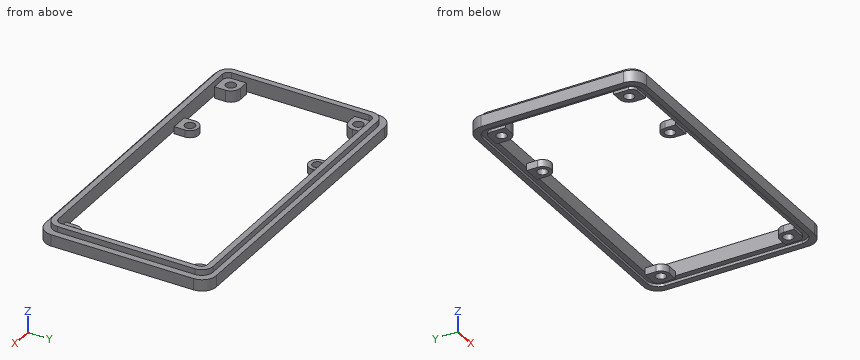
from build123d import *

# Parameters (mm, degrees)
F1_DEPTH = 6
F2_DEPTH = 4
F0_R     = 1.75
F3_DEPTH = 2.5
F4_DEPTH = 4
F5_DEPTH = 1


with BuildPart() as f1:
    # F0 (on Top) → F1 (new body)
    with BuildSketch(Plane.XY):
        with BuildLine():
            Line((48.5, 28), (-48.5, 28))
            ThreePointArc((-48.5, 28), (-51.328427, 26.828427), (-52.5, 24))
            Line((-52.5, 24), (-52.5, -24))
            ThreePointArc((-52.5, -24), (-51.328427, -26.828427), (-48.5, -28))
            Line((-48.5, -28), (48.5, -28))
            ThreePointArc((48.5, -28), (51.328427, -26.828427), (52.5, -24))
            Line((52.5, -24), (52.5, 24))
            ThreePointArc((52.5, 24), (51.328427, 26.828427), (48.5, 28))
        make_face()
        with BuildLine():
            ThreePointArc((-50.5, 24), (-49.914214, 25.414214), (-48.5, 26))
            Line((-48.5, 26), (-43.75, 26))
            Line((-43.75, 26), (-25.9, 26))
            Line((-25.9, 26), (-19.9, 26))
            Line((-19.9, 26), (44.1, 26))
            Line((44.1, 26), (48.5, 26))
            ThreePointArc((48.5, 26), (49.914214, 25.414214), (50.5, 24))
            Line((50.5, 24), (50.5, 19.25))
            Line((50.5, 19.25), (50.5, -19.25))
            Line((50.5, -19.25), (50.5, -24))
            ThreePointArc((50.5, -24), (49.914214, -25.414214), (48.5, -26))
            Line((48.5, -26), (44.1, -26))
            Line((44.1, -26), (-19.9, -26))
            Line((-19.9, -26), (-25.9, -26))
            Line((-25.9, -26), (-43.75, -26))
            Line((-43.75, -26), (-48.5, -26))
            ThreePointArc((-48.5, -26), (-49.914214, -25.414214), (-50.5, -24))
            Line((-50.5, -24), (-50.5, -18.9))
            Line((-50.5, -18.9), (-50.5, 18.9))
            Line((-50.5, 18.9), (-50.5, 24))
        make_face(mode=Mode.SUBTRACT)
    extrude(amount=F1_DEPTH)

    # F0 (on Top) → F2 (join)
    with BuildSketch(Plane.XY):
        with BuildLine():
            Line((49.75, 29.875), (-49.75, 29.875))
            ThreePointArc((-49.75, 29.875), (-53.285534, 28.410534), (-54.75, 24.875))
            Line((-54.75, 24.875), (-54.75, -24.875))
            ThreePointArc((-54.75, -24.875), (-53.285534, -28.410534), (-49.75, -29.875))
            Line((-49.75, -29.875), (49.75, -29.875))
            ThreePointArc((49.75, -29.875), (53.285534, -28.410534), (54.75, -24.875))
            Line((54.75, -24.875), (54.75, 24.875))
            ThreePointArc((54.75, 24.875), (53.285534, 28.410534), (49.75, 29.875))
        make_face()
        with BuildLine():
            ThreePointArc((-52.5, 24), (-51.328427, 26.828427), (-48.5, 28))
            Line((-48.5, 28), (48.5, 28))
            ThreePointArc((48.5, 28), (51.328427, 26.828427), (52.5, 24))
            Line((52.5, 24), (52.5, -24))
            ThreePointArc((52.5, -24), (51.328427, -26.828427), (48.5, -28))
            Line((48.5, -28), (-48.5, -28))
            ThreePointArc((-48.5, -28), (-51.328427, -26.828427), (-52.5, -24))
            Line((-52.5, -24), (-52.5, 24))
        make_face(mode=Mode.SUBTRACT)
    extrude(amount=F2_DEPTH)

    # F0 (on Top) → F3 (join)
    with BuildSketch(Plane.XY):
        with BuildLine():
            Line((-19.9, 26), (-25.9, 26))
            Line((-25.9, 26), (-25.9, 22.25))
            ThreePointArc((-25.9, 22.25), (-22.9, 19.25), (-19.9, 22.25))
            Line((-19.9, 22.25), (-19.9, 26))
        make_face()
        with Locations((-22.9, 22.25)):
            Circle(F0_R, mode=Mode.SUBTRACT)
        with BuildLine():
            Line((48.5, 26), (44.1, 26))
            Line((44.1, 26), (44.1, 22.25))
            ThreePointArc((44.1, 22.25), (44.97868, 20.12868), (47.1, 19.25))
            Line((47.1, 19.25), (50.5, 19.25))
            Line((50.5, 19.25), (50.5, 24))
            ThreePointArc((50.5, 24), (49.914214, 25.414214), (48.5, 26))
        make_face()
        with Locations((47.1, 22.25)):
            Circle(F0_R, mode=Mode.SUBTRACT)
        with BuildLine():
            Line((50.5, -24), (50.5, -19.25))
            Line((50.5, -19.25), (47.1, -19.25))
            ThreePointArc((47.1, -19.25), (44.97868, -20.12868), (44.1, -22.25))
            Line((44.1, -22.25), (44.1, -26))
            Line((44.1, -26), (48.5, -26))
            ThreePointArc((48.5, -26), (49.914214, -25.414214), (50.5, -24))
        make_face()
        with Locations((47.1, -22.25)):
            Circle(F0_R, mode=Mode.SUBTRACT)
        with BuildLine():
            Line((-25.9, -22.25), (-25.9, -26))
            Line((-25.9, -26), (-19.9, -26))
            Line((-19.9, -26), (-19.9, -22.25))
            ThreePointArc((-19.9, -22.25), (-22.9, -19.25), (-25.9, -22.25))
        make_face()
        with Locations((-22.9, -22.25)):
            Circle(F0_R, mode=Mode.SUBTRACT)
    extrude(amount=F3_DEPTH)

    # F0 (on Top) → F4 (join)
    with BuildSketch(Plane.XY):
        with BuildLine():
            Line((-43.75, 26), (-48.5, 26))
            ThreePointArc((-48.5, 26), (-49.914214, 25.414214), (-50.5, 24))
            Line((-50.5, 24), (-50.5, 18.9))
            Line((-50.5, 18.9), (-47.1, 18.9))
            ThreePointArc((-47.1, 18.9), (-44.731192, 19.881192), (-43.75, 22.25))
            Line((-43.75, 22.25), (-43.75, 26))
        make_face()
        with Locations((-47.1, 22.25)):
            Circle(F0_R, mode=Mode.SUBTRACT)
        with BuildLine():
            Line((-47.1, -18.9), (-50.5, -18.9))
            Line((-50.5, -18.9), (-50.5, -24))
            ThreePointArc((-50.5, -24), (-49.914214, -25.414214), (-48.5, -26))
            Line((-48.5, -26), (-43.75, -26))
            Line((-43.75, -26), (-43.75, -22.25))
            ThreePointArc((-43.75, -22.25), (-44.731192, -19.881192), (-47.1, -18.9))
        make_face()
        with Locations((-47.1, -22.25)):
            Circle(F0_R, mode=Mode.SUBTRACT)
    extrude(amount=F4_DEPTH)

    # F0 (on Top) → F5 (cut)
    with BuildSketch(Plane.XY):
        with BuildLine():
            Line((48.5, 28), (-48.5, 28))
            ThreePointArc((-48.5, 28), (-51.328427, 26.828427), (-52.5, 24))
            Line((-52.5, 24), (-52.5, -24))
            ThreePointArc((-52.5, -24), (-51.328427, -26.828427), (-48.5, -28))
            Line((-48.5, -28), (48.5, -28))
            ThreePointArc((48.5, -28), (51.328427, -26.828427), (52.5, -24))
            Line((52.5, -24), (52.5, 24))
            ThreePointArc((52.5, 24), (51.328427, 26.828427), (48.5, 28))
        make_face()
        with BuildLine():
            ThreePointArc((-50.5, 24), (-49.914214, 25.414214), (-48.5, 26))
            Line((-48.5, 26), (-43.75, 26))
            Line((-43.75, 26), (-25.9, 26))
            Line((-25.9, 26), (-19.9, 26))
            Line((-19.9, 26), (44.1, 26))
            Line((44.1, 26), (48.5, 26))
            ThreePointArc((48.5, 26), (49.914214, 25.414214), (50.5, 24))
            Line((50.5, 24), (50.5, 19.25))
            Line((50.5, 19.25), (50.5, -19.25))
            Line((50.5, -19.25), (50.5, -24))
            ThreePointArc((50.5, -24), (49.914214, -25.414214), (48.5, -26))
            Line((48.5, -26), (44.1, -26))
            Line((44.1, -26), (-19.9, -26))
            Line((-19.9, -26), (-25.9, -26))
            Line((-25.9, -26), (-43.75, -26))
            Line((-43.75, -26), (-48.5, -26))
            ThreePointArc((-48.5, -26), (-49.914214, -25.414214), (-50.5, -24))
            Line((-50.5, -24), (-50.5, -18.9))
            Line((-50.5, -18.9), (-50.5, 18.9))
            Line((-50.5, 18.9), (-50.5, 24))
        make_face(mode=Mode.SUBTRACT)
    extrude(amount=F5_DEPTH, mode=Mode.SUBTRACT)


solid = f1.part
The listing builds one solid part. Answer for the finished solid, in the listing's coordinates (mm). Round coordinates to 2 decimals unless told otherwise and drop trailing zeros. Write each loop counter-clockwise with the first axis right and the second up, starting at its lowest first coordinate (ties: lowest second). Pieces come first, ordered by that corner, then holes. Notation, with made-up numbers: (-26.5, 42.25) - (-13.5, 42.25) arc R16 ccw to (-13.5, 70.25) - close; hole circle Ø10 at (24.25, 43). An arc over 180 degrees is marked (long way). Use one line per item in the form item = value. Start each with the question number.
Item 1: A cutting plane is placed at C-C (x = -22.9). Give the number of separate pieces and of enclosed holes in the cut face, plus the area to 4 significant figures.
Item 2: A cutting plane is placed at B-B (y = 14.5). Write down the section's boundary in (x, z).
Item 3: Find the intervals of material crossed by line 1 (X direction, y = -22, z = 3.55); line 2 (Y direction, x = 38, z = 3.75) (3 decimals); line 3 (Y direction, x = -50, z = 1.9), in increasing order. Write a range as [from, to].
Item 4: Flat-ended cylindrical pins translate along their axes: pin 1 Ø3.5 at (x, y) = (-46.5, -24) entering from +Z; pin 2 Ø0.6 at (x, z) = (-21.5, 5.5) entering from -Y. Find the tip coordinate at first contact, or state that the pin passes through.
Item 5: A cutting plane is placed at A-A (x = 19). Write down the section's boundary in (y, z) (3 decimals), plus the area to 3 significant figures.
The answers:
q1.separate_pieces = 4
q1.enclosed_holes = 0
q1.area = 51.25 mm^2
q2.outline = (-54.75, 0) - (-52.5, 0) - (-52.5, 1) - (-50.5, 1) - (-50.5, 6) - (-52.5, 6) - (-52.5, 4) - (-54.75, 4) - close; (50.5, 1) - (52.5, 1) - (52.5, 0) - (54.75, 0) - (54.75, 4) - (52.5, 4) - (52.5, 6) - (50.5, 6) - close
q3.line_1 = [-54.75, -48.83], [-45.37, -43.76], [50.5, 54.75]
q3.line_2 = [-29.875, -26], [26, 29.875]
q3.line_3 = [-29.87, -18.9], [18.9, 29.87]
q4.pin_1 = 4
q4.pin_2 = -28
q5.outline = (-29.875, 0) - (-28, 0) - (-28, 1) - (-26, 1) - (-26, 6) - (-28, 6) - (-28, 4) - (-29.875, 4) - close; (26, 1) - (28, 1) - (28, 0) - (29.875, 0) - (29.875, 4) - (28, 4) - (28, 6) - (26, 6) - close
q5.area = 35.0 mm^2
